from build123d import *

# Parameters (mm, degrees)
F0_R     = 49.15
F0_R_2   = 27.95
F1_DEPTH = 22.25
F2_R     = 10
F3_R     = 5
F7_DEPTH = 2
F9_DEPTH = 20


with BuildPart() as f1:
    # F0 (on Front) → F1 (new body, symmetric)
    with BuildSketch(Plane.XZ):
        with Locations((0, 49.15)):
            Circle(F0_R)
        with Locations((0, 49.15)):
            Circle(F0_R_2, mode=Mode.SUBTRACT)
    extrude(amount=F1_DEPTH, both=True)

    # F2
    f2_edges = [f1.edges().sort_by_distance(p)[0] for p in [
        (-49.15, -22.25, 49.15),
        (-49.15, 22.25, 49.15),
    ]]
    fillet(f2_edges, radius=F2_R)

    # F3
    f3_edges = [f1.edges().sort_by_distance(p)[0] for p in [
        (-27.95, 22.25, 49.15),
        (-27.95, -22.25, 49.15),
    ]]
    fillet(f3_edges, radius=F3_R)



with BuildPart() as f7:
    # F5 (on face) → F7 (new body)
    with BuildSketch(Plane(origin=(0, 0, -9.7), x_dir=(1, 0, 0), z_dir=(0, 0, -1))):
        Polygon((43, 10), (43, -10), (57.4, -10), (60.3, -7.1), (60.3, 7.1), (57.4, 10), align=None)
        with BuildLine():
            ThreePointArc((54.6, 2.8), (56.5798989873, 1.9798989873), (57.4, 0))
            ThreePointArc((57.4, 0), (56.5798989873, -1.9798989873), (54.6, -2.8))
            Line((54.6, -2.8), (50.8, -2.8))
            ThreePointArc((50.8, -2.8), (48, 0), (50.8, 2.8))
            Line((50.8, 2.8), (54.6, 2.8))
        make_face(mode=Mode.SUBTRACT)
    extrude(amount=-F7_DEPTH)


with BuildPart() as f7b:
    # F5 (on face) → F7, piece 2 (new body)
    with BuildSketch(Plane(origin=(0, 0, -9.7), x_dir=(1, 0, 0), z_dir=(0, 0, -1))):
        Polygon((-57.4, -10), (-43, -10), (-43, 10), (-57.4, 10), (-60.3, 7.1), (-60.3, -7.1), align=None)
        with BuildLine():
            ThreePointArc((-54.6, -2.8), (-57.4, 0), (-54.6, 2.8))
            Line((-54.6, 2.8), (-50.8, 2.8))
            ThreePointArc((-50.8, 2.8), (-48.8201010127, 1.9798989873), (-48, 0))
            ThreePointArc((-48, 0), (-48.8201010127, -1.9798989873), (-50.8, -2.8))
            Line((-50.8, -2.8), (-54.6, -2.8))
        make_face(mode=Mode.SUBTRACT)
    extrude(amount=-F7_DEPTH)


with BuildPart() as f1_1:
    add(f1.part)

    add(f7.part)  # F9 merges F7

    add(f7b.part)  # F9 merges F7b
    # F8 (on face) → F9 (join, through all)
    with BuildSketch(Plane(origin=(0, 10, 0), x_dir=(-1, 0, 0), z_dir=(0, 1, 0))):
        with BuildLine():
            Line((43, -7.7), (29.6497265558, 9.9503033791))
            ThreePointArc((29.6497265558, 9.9503033791), (29.1663333729, 9.5893187927), (28.6785456751, 9.2342948458))
            Line((28.6785456751, 9.2342948458), (43, -9.7))
            Line((43, -9.7), (43, -7.7))
        make_face()
        with BuildLine():
            ThreePointArc((-28.6785456751, 9.2342948458), (-29.1663333729, 9.5893187927), (-29.6497265558, 9.9503033791))
            Line((-29.6497265558, 9.9503033791), (-43, -7.7))
            Line((-43, -7.7), (-43, -9.7))
            Line((-43, -9.7), (-28.6785456751, 9.2342948458))
        make_face()
    extrude(amount=-F9_DEPTH)


solid = f1_1.part
Design review of the part built by this model. Coordinates are the model's own, in mm. A direction names the side the tool comes from. Round coordinates to 2 decimals unless told otherwise and drop trailing zeros. Write each loop counter-clockwise with the first axis right and the second up, starting at its lowest first coordinate (ties: lowest second). Pieces come first, ordered by that corner, then holes. Notation, with made-up numbers: (37, 25.25) -> (69, 25.25) arc R11 ccw to (69, 43.25) -> close; hole circle Ø4 at (0.5, -36). An arc over 180 degrees is marked (long way). One line per question, with ' | ' between items.
(1) Take a section at A-A, the plane x = 0. State the section outline as (y, z) points.
Result sheet:
outline: (-22.25, 10) arc R10 ccw to (-12.25, 0) -> (12.25, 0) arc R10 ccw to (22.25, 10) -> (22.25, 16.2) arc R5 ccw to (17.25, 21.2) -> (-17.25, 21.2) arc R5 ccw to (-22.25, 16.2) -> close; (-22.25, 82.1) arc R5 ccw to (-17.25, 77.1) -> (17.25, 77.1) arc R5 ccw to (22.25, 82.1) -> (22.25, 88.3) arc R10 ccw to (12.25, 98.3) -> (-12.25, 98.3) arc R10 ccw to (-22.25, 88.3) -> close
(2) Wall thickness on line 1 (Z direction, x = 0, y = -10); line 2 (X direction, y = 0, z = 49); line 3 (Z direction, x = 12.5, y = -9.5): over which ranges is each line inside the solid? List them lowest first. Write a range as [from, to].
Result sheet:
line 1: [0, 21.2], [77.1, 98.3] | line 2: [-49.15, -27.95], [27.95, 49.15] | line 3: [1.62, 24.15], [74.15, 96.68]
(3) Machinability: for faces 5 (the flat face through (36.23, 0.14, 1.25)), 6 (the flat face through (41, -10, -6)), 7 (the flat face through (-48, 2, -7.7)), 8 (the flat face through (-35.74, 0.14, -0.1)), 9 (the flat face through (41, 10, -6)), which of the approach directions +Z, -Z, +X, -X, +Y, -Y give a long, thin tool a straight path to every point of the face, cutting with its end or side? Answer none if there is none.
Result sheet:
face 5: +X, +Y, -Y | face 6: -Z, +X, -Y | face 7: -X, +Y, -Y | face 8: -Z, +Y, -Y | face 9: -Z, +X, +Y
(4) Take a section at C-C, the plane z = 4.5. State how many separate pieces and enclosed holes the cut face has, and give its area (3 significant figures).
Result sheet:
separate pieces: 3 | enclosed holes: 0 | area: 1,620 mm2
(5) Take a section at D-D, the plane y = -15. State the section outline as (x, z) points, and give its area (3 significant figures).
Result sheet:
outline: circle Ø97.53 at (0, 49.15); hole circle Ø55.9 at (0, 49.15) | area: 5,020 mm2
(6) Take a section at B-B, the plane z = 49.15. State the section outline as (x, y) points.
Result sheet:
outline: (-49.15, -12.25) arc R10 ccw to (-39.15, -22.25) -> (-32.95, -22.25) arc R5 ccw to (-27.95, -17.25) -> (-27.95, 17.25) arc R5 ccw to (-32.95, 22.25) -> (-39.15, 22.25) arc R10 ccw to (-49.15, 12.25) -> close; (27.95, -17.25) arc R5 ccw to (32.95, -22.25) -> (39.15, -22.25) arc R10 ccw to (49.15, -12.25) -> (49.15, 12.25) arc R10 ccw to (39.15, 22.25) -> (32.95, 22.25) arc R5 ccw to (27.95, 17.25) -> close
(7) Draft analysis for pull direction X (two halves, no side actions). For faces 1 (the flat face through (-41, 10, -6)), 2 (the flat face through (-36.42, 0.14, 1)), 3 (the cylindrical face through (-10.655, -0.172, 1.169)), 4 (the cylindrical face through (-6.059, 0.241, 21.865)), state which applies: released by +X, released by -X, zero draft, split by the parting line, or undercut.
Result sheet:
face 1: zero draft | face 2: released by -X | face 3: undercut | face 4: undercut
(8) Insertion check: P1, Ø6, axis at y = 2, z = 56.5, coming from the +X side; P2, Ø8, axis at x = 28.5, y = 9.5, coming from the -Z side; P3, Ø15.5, axis at x = -45.5, z = 2.5, coming from the -Y side; P4, Ø3, axis at y = -8.5, z = 56, coming from the -X side. Each pin has a flat end and moves straight along its axis. Give the tip position at first contact, or say it passes through.
Result sheet:
P1: x = 48.96 | P2: z = 4.18 | P3: through | P4: x = -48.86
